Check sheet for the drawn part. Datum: minimum x, y, z corner. Units: mm. A direction names the side the tool comes from. Give positions to 0.01 mm unless a question says otherwise; leave off trailing zeros. Write each loop counter-clockwise with the first axis right and the second up, starting at its lowest first coordinate (ties: lowest second). Pieces come first, ordered by that corner, then holes. Notation, with made-up numbers: (33.5, 76.5) - (70.5, 76.5) arc R22 cw to (70.5, 82.5) - close; hole circle Ø7 at (41.5, 25). An arc over 180 degrees is marked (long way). Answer as a JSON object with one key per item and string values. Group by question number.
Item 1: Go/stop test with a flat-tipped pin: pin 1 (4 mm diameter, centred on x = 22, y = 7, fed in from -Z). Record where the tip stops, or that it passes through.
Item 2: Tool access check on the marked faces 1 and 2. Record the directions out of +Z, -Z, +X, -X, +Y, -Y that give a thin tool (end or side, any length) a straight path to the whole face; none if there is none.
Item 3: Sectioned sample at A-A, the plane z = 0.5. Record the boundary of the cut face in (x, y), and give its area (3 significant figures).
Item 4: Sectioned sample at B-B, the plane y = 29.5. Record the boundary of the cut face in (x, z), and give its area (3 significant figures).
Item 5: Scan lines: line 1 along X through (y, z) = (39, 1.6); line 2 along Y through (x, z) = (10.5, 1.6); line 3 along Z through (x, y) = (24, 46.5). Record each from-to range of solid material in increasing order. Write a range as [from, to].
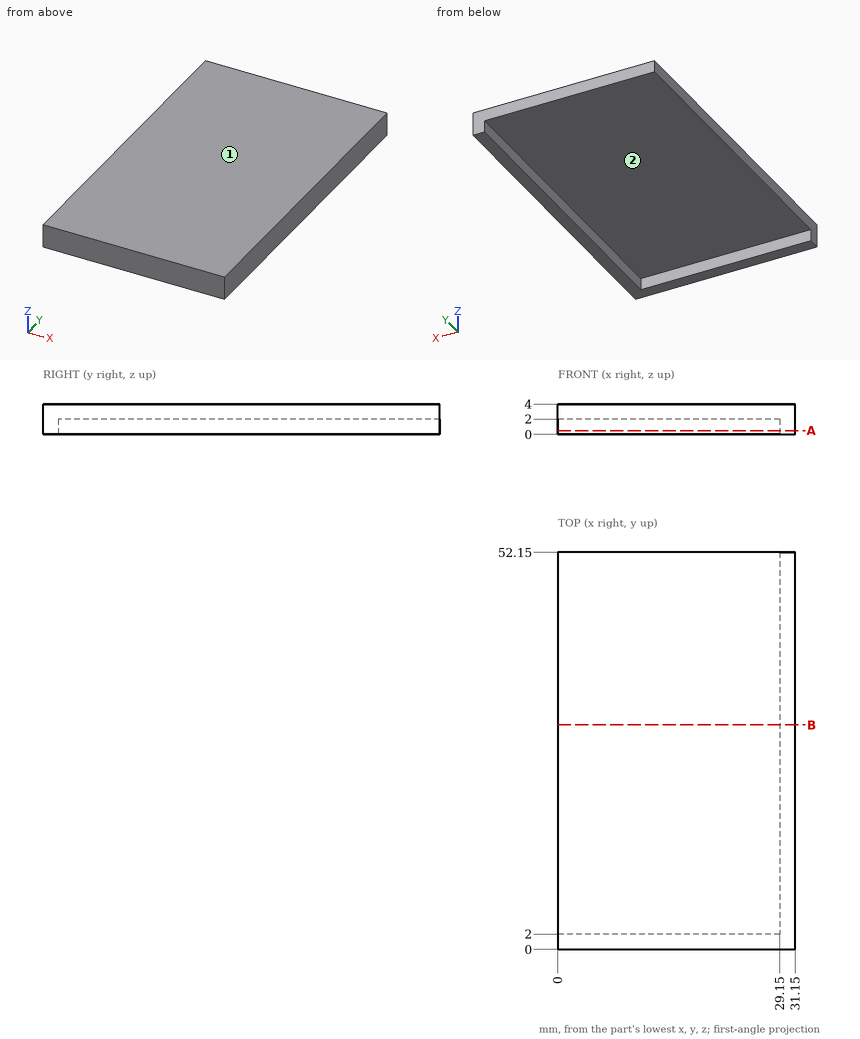
Geometry check:
{
 "1": {"pin 1": "z = 2"},
 "2": {"face 1": "+Z, +X, -X, +Y, -Y", "face 2": "-Z, -X, +Y"},
 "3": {"outline": "(0, 0) - (31.15, 0) - (31.15, 52.15) - (29.15, 52.15) - (29.15, 2) - (0, 2) - close", "area": "163 mm^2"},
 "4": {"outline": "(0, 2) - (29.15, 2) - (29.15, 0) - (31.15, 0) - (31.15, 4) - (0, 4) - close", "area": "66.3 mm^2"},
 "5": {"line 1": "[29.15, 31.15]", "line 2": "[0, 2]", "line 3": "[2, 4]"}
}
